The model under review builds one solid part; all positions refer to its coordinate system, in mm. A direction names the side the tool comes from. Round coordinates to 2 decimals unless told otherwise and drop trailing zeros. Write each loop counter-clockwise with the first axis right and the second up, starting at its lowest first coordinate (ties: lowest second). Pieces come first, ordered by that corner, then holes. Notation, with made-up numbers: M 40.25,38 L 86.25,38 A15 cw 86.25,59 Z; hole C 60,83.5 d2. An arc over 180 degrees is marked long. Write item = value, one per line. Start each with the question number.
Item 1: Take a section at D-D, the plane x = 8. Give the boundary of the cut face in (y, z).
Item 2: The part is to be moulded in two halves that separate along X. For faces 5 (the flat face through (0, 12, 9)), 6 (the flat face through (19, 8, 13.5)), 7 (the flat face through (-52.5, 6, 17)), say which applies: +X half, -X half, draft (parallel to the pull), parting line (faces both ways), or undercut.
Item 3: Take a section at A-A, the plane z = 5. Give the boundary of the cut face in (x, y).
Item 4: Tool access review of faces 1 (the flat face through (0, 4, 17)), 2 (the flat face through (17, 8, 2)), 3 (the flat face through (-37, 8, 28.55)), 4 (the cylindrical face through (-42.479, 4.407, 17.117)): name each direction out of +Z, -Z, +X, -X, +Y, -Y from which nothing blocks a thin tool from reaching the whole face with its end or side.
Item 5: To check wall thickness, follow line 1 along X through (y, z) = (10.5, 5); line 2 along X through (y, z) = (7.5, 5); line 3 along X through (y, z) = (4.25, 4.5). State the ranges of each line that lie inside material, in increasing order.
Item 6: Take a section at C-C, the plane y = -5. Give the boundary of the cut face in (x, z).
Item 7: Take a section at B-B, the plane x = 38. Give the boundary of the cut face in (y, z).
Item 8: For pin 1 Ø4 at (x, z) = (-11.5, 30) entering from -Y; pin 2 Ø4 at (x, z) = (9.5, 21) entering from +Y; pin 3 Ø12 at (x, z) = (20.5, 31) entering from -Y, all flat-tipped, find the tip position at first contact; note any pin that passes through.
from build123d import *

# Parameters (mm, degrees)
EXTRUDE_1_DEPTH     = 34.55
SKETCH_2_W          = 40
SKETCH_2_H          = 8
CUT_EXTRUDE_1_DEPTH = 16
CUT_EXTRUDE_2_DEPTH = 10
SKETCH_4_W          = 10.1
SKETCH_4_H          = 5.2
CUT_EXTRUDE_3_DEPTH = 10
CHAMFER_1_SIZE      = 2
CHAMFER_2_SIZE      = 1
SKETCH_6_R          = 1.6
EXTRUDE_2_DEPTH     = 6.9
SKETCH_7_R          = 1.6
CUT_EXTRUDE_4_DEPTH = 10
SKETCH_8_R          = 1.6
EXTRUDE_3_DEPTH     = 5.5
SKETCH_10_W         = 40
SKETCH_10_H         = 10
CUT_EXTRUDE_5_DEPTH = 2
CUT_EXTRUDE_6_DEPTH = 10
SKETCH_12_W         = 34
SKETCH_12_H         = 2.5
CUT_EXTRUDE_7_DEPTH = 4.9
EXTRUDE_START       = -6
EXTRUDE_4_DEPTH     = 22.55
FILLET_1_R          = 1


with BuildPart() as part:
    # 草图1 → 凸台-拉伸1 (new body)
    with BuildSketch(Plane.XY):
        Polygon((0, 0), (22.5, 0), (22.5, 12), (-22.5, 12), (-22.5, 0), align=None)
    extrude(amount=EXTRUDE_1_DEPTH)

    # 草图2 → 切除-拉伸1 (cut)
    with BuildSketch(Plane.XY.offset(34.55)):
        with Locations((0, 8)):
            Rectangle(SKETCH_2_W, SKETCH_2_H)
    extrude(amount=-CUT_EXTRUDE_1_DEPTH, mode=Mode.SUBTRACT)

    # 草图3 → 切除-拉伸2 (cut)
    with BuildSketch(Plane.XZ):
        Polygon((0, 2), (20, 2), (20, 17), (-20, 17), (-20, 2), align=None)
    extrude(amount=-CUT_EXTRUDE_2_DEPTH, mode=Mode.SUBTRACT)

    # 草图4 → 切除-拉伸3 (cut)
    with BuildSketch(Plane.XY.offset(18.55)):
        with Locations((-8.99, 7.8)):
            Rectangle(SKETCH_4_W, SKETCH_4_H)
        with Locations((8.99, 7.8)):
            Rectangle(SKETCH_4_W, SKETCH_4_H)
    extrude(amount=-CUT_EXTRUDE_3_DEPTH, mode=Mode.SUBTRACT)

    # 倒角1
    chamfer_1_edges = [part.edges().sort_by_distance(p)[0] for p in [
        (20, 4, 26.55),
        (-20, 4, 26.55),
    ]]
    chamfer(chamfer_1_edges, length=CHAMFER_1_SIZE)

    # 倒角2
    chamfer_2_edges = [part.edges().sort_by_distance(p)[0] for p in [
        (-8.99, 10.4, 18.55),
        (-14.04, 7.8, 18.55),
        (-8.99, 5.2, 18.55),
        (-3.94, 7.8, 18.55),
        (3.94, 7.8, 18.55),
        (8.99, 5.2, 18.55),
        (14.04, 7.8, 18.55),
        (8.99, 10.4, 18.55),
    ]]
    chamfer(chamfer_2_edges, length=CHAMFER_2_SIZE)

    # 草图6 → 凸台-拉伸2 (add)
    with BuildSketch(Plane(origin=(0, 12, 0), x_dir=(1, 0, 0), z_dir=(0, 1, 0))):
        with BuildLine():
            Line((22.5, 0), (22.5, -13.5))
            Line((22.5, -13.5), (17, -13.5))
            ThreePointArc((17, -13.5), (15.232233047, -12.767766953), (14.5, -11))
            Line((14.5, -11), (14.5, -5))
            Line((14.5, -5), (14.5, 0))
            Line((14.5, 0), (22.5, 0))
        make_face()
        with Locations((17, -5)):
            Circle(SKETCH_6_R, mode=Mode.SUBTRACT)
        with Locations((17, -11)):
            Circle(SKETCH_6_R, mode=Mode.SUBTRACT)
        with BuildLine():
            Line((-14.5, 0), (-22.5, 0))
            Line((-22.5, 0), (-22.5, -13.5))
            Line((-22.5, -13.5), (-17, -13.5))
            ThreePointArc((-17, -13.5), (-15.232233047, -12.767766953), (-14.5, -11))
            Line((-14.5, -11), (-14.5, -5))
            Line((-14.5, -5), (-14.5, 0))
        make_face()
        with Locations((-17, -11)):
            Circle(SKETCH_6_R, mode=Mode.SUBTRACT)
        with Locations((-17, -5)):
            Circle(SKETCH_6_R, mode=Mode.SUBTRACT)
    extrude(amount=-EXTRUDE_2_DEPTH)

    # 草图7 → 切除-拉伸4 (cut)
    with BuildSketch(Plane(origin=(0, 12, 0), x_dir=(1, 0, 0), z_dir=(0, 1, 0))):
        with Locations((17, -5)):
            Circle(SKETCH_7_R)
        with Locations((17, -11)):
            Circle(SKETCH_7_R)
        with Locations((-17, -5)):
            Circle(SKETCH_7_R)
        with Locations((-17, -11)):
            Circle(SKETCH_7_R)
    extrude(amount=-CUT_EXTRUDE_4_DEPTH, mode=Mode.SUBTRACT)

    # 草图8 → 凸台-拉伸3 (add)
    with BuildSketch(Plane.XY.offset(34.55)):
        with BuildLine():
            Line((1.843049286, -25.367101461), (9.230566594, -19.615105309))
            ThreePointArc((9.230566594, -19.615105309), (9.814108465, -18.625953935), (10.421644381, -17.651355727))
            Line((10.421644381, -17.651355727), (5.476763257, -11.300448334))
            ThreePointArc((5.476763257, -11.300448334), (6.699551666, -1.476763257), (16.523236743, -2.699551666))
            Line((16.523236743, -2.699551666), (19.967990067, -6.846461039))
            ThreePointArc((19.967990067, -6.846461039), (22.224318463, -5.085470923), (24.58365332, -3.465087309))
            ThreePointArc((24.58365332, -3.465087309), (26.278709649, -3.148232211), (27.365383934, -1.809295278))
            ThreePointArc((27.365383934, -1.809295278), (28.658809968, -1.124546474), (29.972928279, -0.480399834))
            ThreePointArc((29.972928279, -0.480399834), (29.349734714, 1.46572665), (28, 3))
            Line((28, 3), (22.5, 3))
            Line((22.5, 3), (22.5, 4))
            Line((22.5, 4), (-22.5, 4))
            Line((-22.5, 4), (-22.5, 3))
            Line((-22.5, 3), (-28, 3))
            ThreePointArc((-28, 3), (-29.349734714, 1.46572665), (-29.972928279, -0.480399834))
            ThreePointArc((-29.972928279, -0.480399834), (-28.658809968, -1.124546474), (-27.365383934, -1.809295278))
            ThreePointArc((-27.365383934, -1.809295278), (-26.278709649, -3.148232211), (-24.58365332, -3.465087309))
            ThreePointArc((-24.58365332, -3.465087309), (-22.224318463, -5.085470923), (-19.967990067, -6.846461039))
            Line((-19.967990067, -6.846461039), (-16.523236743, -2.699551666))
            ThreePointArc((-16.523236743, -2.699551666), (-6.699551666, -1.476763257), (-5.476763257, -11.300448334))
            Line((-5.476763257, -11.300448334), (-10.421644381, -17.651355727))
            ThreePointArc((-10.421644381, -17.651355727), (-9.814108465, -18.625953935), (-9.230566594, -19.615105309))
            Line((-9.230566594, -19.615105309), (-1.843049286, -25.367101461))
            ThreePointArc((-1.843049286, -25.367101461), (0, -26), (1.843049286, -25.367101461))
        make_face()
        with Locations((25, -1)):
            Circle(SKETCH_8_R, mode=Mode.SUBTRACT)
        with Locations((0, -23)):
            Circle(SKETCH_8_R, mode=Mode.SUBTRACT)
        with Locations((-25, -1)):
            Circle(SKETCH_8_R, mode=Mode.SUBTRACT)
    extrude(amount=-EXTRUDE_3_DEPTH)

    # 草图10 → 切除-拉伸5 (cut)
    with BuildSketch(Plane(origin=(0, 0, 0), x_dir=(-1, 0, 0), z_dir=(0, 0, -1))):
        with Locations((0, 5)):
            Rectangle(SKETCH_10_W, SKETCH_10_H)
    extrude(amount=-CUT_EXTRUDE_5_DEPTH, mode=Mode.SUBTRACT)

    # 草图11 → 切除-拉伸6 (cut)
    with BuildSketch(Plane(origin=(0, 0, 29.05), x_dir=(-1, 0, 0), z_dir=(0, 0, -1))):
        Polygon((-4, -7), (4, -7), (10.421644381, -17.651355727), (10.421644381, -27.0891889), (-10.421644381, -27.0891889), (-10.421644381, -17.651355727), align=None)
    extrude(amount=-CUT_EXTRUDE_6_DEPTH, mode=Mode.SUBTRACT)

    # 草图12 → 切除-拉伸7 (cut)
    with BuildSketch(Plane.XZ.offset(-5.1)):
        with Locations((0, 12.25)):
            Rectangle(SKETCH_12_W, SKETCH_12_H)
    extrude(amount=-CUT_EXTRUDE_7_DEPTH, mode=Mode.SUBTRACT)

    # 草图14 → 凸台-拉伸4 (add)
    with BuildSketch(Plane(origin=(0, 0, 0), x_dir=(-1, 0, 0), z_dir=(0, 0, -1)).offset(EXTRUDE_START)):
        with BuildLine():
            Line((-22.5, 9.5), (-52.5, 9.5))
            Line((-52.5, 9.5), (-52.5, 2.932014979))
            ThreePointArc((-52.5, 2.932014979), (-42.310755549, 2.352789548), (-32.5, -0.458843457))
            Line((-32.5, -0.458843457), (-32.5, 3))
            Line((-32.5, 3), (-22.5, 3))
            Line((-22.5, 3), (-22.5, 9.5))
        make_face()
        with BuildLine():
            Line((-24.5, 7.5), (-50.5, 7.5))
            Line((-50.5, 7.5), (-50.5, 4.997395763))
            ThreePointArc((-50.5, 4.997395763), (-42.390809061, 4.393039713), (-34.5, 2.428515274))
            Line((-34.5, 2.428515274), (-34.5, 5))
            Line((-34.5, 5), (-24.5, 5))
            Line((-24.5, 5), (-24.5, 7.5))
        make_face(mode=Mode.SUBTRACT)
        with BuildLine():
            Line((32.5, 3), (32.5, -0.458843457))
            ThreePointArc((32.5, -0.458843457), (42.310755549, 2.352789548), (52.5, 2.932014979))
            Line((52.5, 2.932014979), (52.5, 9.5))
            Line((52.5, 9.5), (22.5, 9.5))
            Line((22.5, 9.5), (22.5, 3))
            Line((22.5, 3), (32.5, 3))
        make_face()
        with BuildLine():
            Line((34.5, 5), (34.5, 2.428515274))
            ThreePointArc((34.5, 2.428515274), (42.390809061, 4.393039713), (50.5, 4.997395763))
            Line((50.5, 4.997395763), (50.5, 7.5))
            Line((50.5, 7.5), (24.5, 7.5))
            Line((24.5, 7.5), (24.5, 5))
            Line((24.5, 5), (34.5, 5))
        make_face(mode=Mode.SUBTRACT)
    extrude(amount=-EXTRUDE_4_DEPTH)

    # 圆角1
    fillet_1_edges = [part.edges().sort_by_distance(p)[0] for p in [
        (32.5, 3, 17.275),
        (32.5, -0.458843457, 17.275),
        (52.5, 2.932014979, 17.275),
        (52.5, 9.5, 17.275),
        (24.5, 5, 17.275),
        (34.5, 5, 17.275),
        (34.5, 2.428515274, 17.275),
        (50.5, 4.997395763, 17.275),
        (50.5, 7.5, 17.275),
        (24.5, 7.5, 17.275),
        (-52.5, 2.932014979, 17.275),
        (-32.5, -0.458843457, 17.275),
        (-32.5, 3, 17.275),
        (-52.5, 9.5, 17.275),
        (-24.5, 5, 17.275),
        (-24.5, 7.5, 17.275),
        (-50.5, 7.5, 17.275),
        (-50.5, 4.997395763, 17.275),
        (-34.5, 2.428515274, 17.275),
        (-34.5, 5, 17.275),
    ]]
    fillet(fillet_1_edges, radius=FILLET_1_R)


solid = part.part
Response values:
q1.outline = M -0.68,29.05 L 0,29.05 L 0,17 L 5.2,17 L 5.2,17.55 L 4.2,18.55 L 4,18.55 L 4,34.55 L -0.68,34.55 Z; M 10,0 L 12,0 L 12,18.55 L 11.4,18.55 L 10.4,17.55 L 10.4,8.55 L 10,8.55 Z
q2.face_5 = draft
q2.face_6 = undercut
q2.face_7 = -X half
q3.outline = M -22.5,0 L -20,0 L -20,5.1 L -18.6,5.1 L -18.6,12 L -22.5,12 Z; M -15.4,5.1 L -14.5,5.1 L -14.5,10 L 14.5,10 L 14.5,5.1 L 15.4,5.1 L 15.4,12 L -15.4,12 Z; M 18.6,5.1 L 20,5.1 L 20,0 L 22.5,0 L 22.5,12 L 18.6,12 Z
q4.face_1 = -Y
q4.face_2 = -Z, -Y
q4.face_3 = +Z, -X, +Y, -Y
q4.face_4 = +Z, -Z
q5.line_1 = -22.5 to -18.6, -15.4 to 15.4, 18.6 to 22.5
q5.line_2 = -22.5 to -18.6, -15.4 to -14.5, 14.5 to 15.4, 18.6 to 22.5
q5.line_3 = -22.5 to -20, 20 to 22.5
q6.outline = M -22.34,29.05 L -18.43,29.05 L -18.43,34.55 L -22.34,34.55 Z; M -4.29,29.05 L 4.29,29.05 L 4.29,34.55 L -4.29,34.55 Z; M 18.43,29.05 L 22.34,29.05 L 22.34,34.55 L 18.43,34.55 Z
q7.outline = M 1.41,6 L 3.48,6 L 3.48,28.55 L 1.41,28.55 Z; M 7.5,6 L 9.5,6 L 9.5,28.55 L 7.5,28.55 Z
q8.pin_1 = -0.46
q8.pin_2 = 4
q8.pin_3 = -6.85
